Geometry: final body of the model. Coordinates: model frame, mm. A direction names the side the tool comes from. Give positions to 0.01 mm unless a question says otherwise; leave off trailing zeros. Loops run counter-clockwise (first coordinate to the right, second up) from the corner with the lowest first, then second, coordinate; pieces in that order, holes last. Notation, with made-up numbers: (12, 60) - (17, 60) arc R32 ccw to (17, 88) - close; hole circle Ø3 at (84.25, 24.5). An arc over 180 degrees is marked (long way). Use one line per item in the form item = value.
```python
from build123d import *

# Parameters (mm, degrees)
BOSS_EXTRUDE1_DEPTH = 70.9
SKETCH6_W           = 5
SKETCH6_H           = 70.9
BOSS_EXTRUDE2_DEPTH = 4
LPATTERN1_COUNT     = 6
LPATTERN1_PITCH     = 20


with BuildPart() as part:
    # Sketch1 → Boss-Extrude1 (new body)
    with BuildSketch(Plane.XY):
        with BuildLine():
            Line((-2.334965582, 3.503489658), (97.520200597, 70.053814883))
            ThreePointArc((97.520200597, 70.053814883), (103.358655837, 68.885290806), (102.19013176, 63.046835566))
            Line((102.19013176, 63.046835566), (2.334965582, -3.503489658))
            ThreePointArc((2.334965582, -3.503489658), (-3.503489658, -2.334965582), (-2.334965582, 3.503489658))
        make_face()
        with BuildLine():
            Line((-1.996509757, 2.995654985), (97.858656422, 69.54598021))
            ThreePointArc((97.858656422, 69.54598021), (102.850821164, 68.546834981), (101.851675935, 63.554670239))
            Line((101.851675935, 63.554670239), (1.996509757, -2.995654985))
            ThreePointArc((1.996509757, -2.995654985), (-2.995654985, -1.996509757), (-1.996509757, 2.995654985))
        make_face(mode=Mode.SUBTRACT)
    extrude(amount=BOSS_EXTRUDE1_DEPTH)

    # Sketch6 → Boss-Extrude2 (add)
    with BuildSketch(Plane(origin=(-2.334965582, 3.503489658, 0), x_dir=(0.8321263848202342, 0.554586043536986, 0), z_dir=(-0.554586043536986, 0.8321263848202342, 0))):
        with Locations((8.653433918, -35.45)):
            Rectangle(SKETCH6_W, SKETCH6_H)
    boss_extrude2 = extrude(amount=BOSS_EXTRUDE2_DEPTH)

    # LPattern1: Boss-Extrude2 ×6
    with Locations(*[Vector(0.8321263848202339, 0.5545860435369864, 0) * (i * LPATTERN1_PITCH) for i in range(1, LPATTERN1_COUNT)]):
        add(boss_extrude2)


solid = part.part
```
(1) Pull-direction query (Y, two-part tool) for faces 5 (the face through (84.9, 64.02, 35.95)), 6 (the face through (79.67, 58.157, 34.954)), 7 (the face through (52.55, 44.89, 34.95)), 8 (the face through (54, 42, 0)); classes: released by +Y, released by -Y, zero draft, split by the parting line, or undercut.
Solution:
face_5 = undercut
face_6 = undercut
face_7 = released by +Y
face_8 = zero draft
(2) Material intervals for L1, parallel to Y at x = 2.5, z = 8.5; L2, parallel to X at y = 67.5, z = 15; L3, parallel to X at y = 56, z = 15.5, sorted ascending. Write a range as from..to.
Solution:
L1 = -3.39..-2.66, 5.99..6.73, 7.34..11.53
L2 = 86.48..88.59, 93.69..94.79, 103.33..103.96
L3 = 69.22..72.22, 76.43..77.53, 90.52..91.62
(3) Cut plane B-B (y = 27.5). Return the cut outline in (x, z), plus the area to 3 significant figures.
Solution:
outline = (33.67, 0) - (34.77, 0) - (34.77, 70.9) - (33.67, 70.9) - close; (47.75, 0) - (48.85, 0) - (48.85, 70.9) - (47.75, 70.9) - close
area = 156 mm2
(4) Pin query (flat end, axial travel): P1, Ø6, axis at y = 42.5, z = 13.5, coming from the +X side; P2, Ø1.5, axis at y = 31.5, z = 59, coming from the +X side; P3, Ø3, axis at y = 17.5, z = 43, coming from the +X side. Return the tip coordinate at first contact, or that it passes through.
Solution:
P1 = 75.86
P2 = 55.98
P3 = 36.1
(5) Cut plane C-C (x = 82). Return the cut outline in (y, z), plus the area to 3 significant figures.
Solution:
outline = (49.59, 0) - (50.32, 0) - (50.32, 70.9) - (49.59, 70.9) - close; (58.98, 0) - (59.71, 0) - (59.71, 70.9) - (58.98, 70.9) - close
area = 104 mm2
(6) Access query for faces 1 (the face through (93.79, 67.57, 34.95)), 2 (the face through (52.623, 30.745, 34.954)), 3 (the face through (18.334, 19.649, 35.946)), 4 (the face through (69.19, 55.98, 34.95)). Directions: +Z, -Z, +X, -X, +Y, -Y. A direction counts if a zero-diameter tool reaches every point of the face in a straight line with its end or side. Return the directions, or none.
Solution:
face_1 = +Z, -Z, +Y
face_2 = +Z, -Z
face_3 = +Z, -Z, -X
face_4 = +Z, -Z, -X, +Y
